Could you check a few things on this model? Use its own coordinates, in mm. A direction names the side the tool comes from. Round coordinates to 2 decimals unless told otherwise and drop trailing zeros. Write each loop counter-clockwise with the first axis right and the second up, starting at its lowest first coordinate (ties: lowest second). Pieces come first, ordered by that corner, then holes. Notation, with made-up numbers: M 0.25,38 L 13.25,38 A31 ccw 13.25,63 Z; hole C -14,24 d10. An arc over 180 degrees is marked long. One line per item, written item: value. Start each with the question number.
(1) I want a section at D-D on z = 43.5. Please give me the cut outline in (x, y) (1 decimal).
(2) If I drill on L1, parallel to Y at x = 0, z = 56; L2, parallel to X at y = -0.5, z = 60; L3, parallel to Y at x = -10, z = 33.5, over which ranges is the centre line in solid material (lowest first)?
(3) I want a section at A-A on y = 0. Please give me the cut outline in (x, z) (3 decimals), and give its area (3 significant figures).
(4) Thinking about a two-plate mould opening in X: for faces 1 (the face through (-16.653, 0.733, 34.436)), 2 (the face through (-9.945, 9.12, 60.458)), 3 (the face through (34.131, 0, 21)), which applies, released by +X, released by -X, zero draft, split by the parting line, or undercut?
(5) I want a section at B-B on x = -7. Please give me the cut outline in (y, z), and give its area (3 significant figures).
(6) Which directions (+Z, -Z, +X, -X, +Y, -Y) give clear straight access to the entire face, cutting with the end or side of a thin tool? Please do faces 4 (the face through (20.619, 14.055, 25.964)), 5 (the face through (14, 0, 0)), 6 (the face through (12, -5, 50.8)), 7 (the face through (12, 5, 19.05)).
(7) I'm going to push flat-ended pins straight in: pin 1 Ø8 at (x, z) = (22.5, 52.5) entering from +Y; pin 2 Ø8 at (y, z) = (-1, 13) entering from -X; pin 3 Ø2 at (y, z) = (-3.5, 39) entering from -X; pin 4 Ø1 at (y, z) = (12.5, 62.5) entering from -X. Where does each tip first touch, or does it pass through?
(8) I want a section at C-C on z = 12.5. Please give me the cut outline in (x, y), and give its area (3 significant figures).
```python
from build123d import *

# Parameters (mm, degrees)
SKETCH1_R           = 16.66875
BOSS_EXTRUDE1_DEPTH = 69.85
SKETCH2_R           = 16.66875
BOSS_EXTRUDE2_DEPTH = 34.13125
SKETCH3_R           = 12.7
CUT_EXTRUDE1_DEPTH  = 30.48
SKETCH5_R           = 12.7
CUT_EXTRUDE3_DEPTH  = 80.509822998
SKETCH7_R           = 13.49375
CUT_EXTRUDE4_DEPTH  = 19.05
SKETCH8_R           = 13.49375
CUT_EXTRUDE5_DEPTH  = 19.05
CUT_EXTRUDE6_START  = -19.05
SKETCH9_R           = 13.49375
CUT_EXTRUDE6_DEPTH  = 19.05


with BuildPart() as part:
    # Sketch1 → Boss-Extrude1 (new body)
    with BuildSketch(Plane.XY):
        Circle(SKETCH1_R)
    extrude(amount=BOSS_EXTRUDE1_DEPTH)

    # Sketch2 → Boss-Extrude2 (add)
    with BuildSketch(Plane(origin=(0, 0, 0), x_dir=(0, 0, -1), z_dir=(1, 0, 0))):
        with Locations((-34.925, 0)):
            Circle(SKETCH2_R)
    extrude(amount=BOSS_EXTRUDE2_DEPTH)

    # Sketch3 → Cut-Extrude1 (cut)
    with BuildSketch(Plane(origin=(34.13125, 0, 0), x_dir=(0, 0, -1), z_dir=(1, 0, 0))):
        with Locations((-34.925, 0)):
            Circle(SKETCH3_R)
    extrude(amount=-CUT_EXTRUDE1_DEPTH, mode=Mode.SUBTRACT)

    # Sketch5 → Cut-Extrude3 (cut, through all)
    with BuildSketch(Plane(origin=(0, 0, 0), x_dir=(-1, 0, 0), z_dir=(0, 0, -1))):
        Circle(SKETCH5_R)
    extrude(amount=-CUT_EXTRUDE3_DEPTH, mode=Mode.SUBTRACT)

    # Sketch7 → Cut-Extrude4 (cut)
    with BuildSketch(Plane.XY.offset(69.85)):
        Circle(SKETCH7_R)
    extrude(amount=-CUT_EXTRUDE4_DEPTH, mode=Mode.SUBTRACT)

    # Sketch8 → Cut-Extrude5 (cut)
    with BuildSketch(Plane(origin=(34.13125, 0, 0), x_dir=(0, 0, -1), z_dir=(1, 0, 0))):
        with Locations((-34.925, 0)):
            Circle(SKETCH8_R)
    extrude(amount=-CUT_EXTRUDE5_DEPTH, mode=Mode.SUBTRACT)

    # Sketch9 → Cut-Extrude6 (cut)
    with BuildSketch(Plane(origin=(0, 0, 0), x_dir=(-1, 0, 0), z_dir=(0, 0, -1)).offset(CUT_EXTRUDE6_START)):
        with Locations(Location((0, 0, 0), (0, 0, 180))):
            Circle(SKETCH9_R)
    extrude(amount=CUT_EXTRUDE6_DEPTH, mode=Mode.SUBTRACT)


solid = part.part
```
Found:
1. outline: M 8.6,-14.3 L 34.1,-14.3 L 34.1,-10.4 L 15.1,-10.4 L 15.1,-9.4 L 8.6,-9.4 A12.7 cw long 8.6,9.4 L 15.1,9.4 L 15.1,10.4 L 34.1,10.4 L 34.1,14.3 L 8.6,14.3 A16.7 ccw long Z
2. L1: y = -16.67 to -13.49, 13.49 to 16.67
2. L2: x = -16.66 to -13.48, 13.48 to 16.66
2. L3: y = -13.34 to -7.83, 7.83 to 13.34
3. outline: M -16.669,0 L -13.494,0 L -13.494,19.05 L -12.7,19.05 L -12.7,50.8 L -13.494,50.8 L -13.494,69.85 L -16.669,69.85 Z; M 12.7,19.05 L 13.494,19.05 L 13.494,0 L 16.669,0 L 16.669,18.256 L 34.131,18.256 L 34.131,21.431 L 15.081,21.431 L 15.081,22.225 L 12.7,22.225 Z; M 12.7,47.625 L 15.081,47.625 L 15.081,48.419 L 34.131,48.419 L 34.131,51.594 L 16.669,51.594 L 16.669,69.85 L 13.494,69.85 L 13.494,50.8 L 12.7,50.8 Z
3. area: 502 mm²
4. face 1: split by the parting line
4. face 2: undercut
4. face 3: released by +X
5. outline: M -15.13,0 L -11.54,0 L -11.54,19.05 L -10.6,19.05 L -10.6,50.8 L -11.54,50.8 L -11.54,69.85 L -15.13,69.85 Z; M 10.6,19.05 L 11.54,19.05 L 11.54,0 L 15.13,0 L 15.13,69.85 L 11.54,69.85 L 11.54,50.8 L 10.6,50.8 Z
5. area: 561 mm²
6. face 4: +X
6. face 5: -Z, +X, -X, +Y, -Y
6. face 6: +Z
6. face 7: -Z
7. pin 1: stops at y = 9.67
7. pin 2: stops at x = -16.67
7. pin 3: stops at x = -16.48
7. pin 4: stops at x = -11.57
8. outline: C 0,0 d33.34; hole C 0,0 d26.99
8. area: 301 mm²
